The listing builds one solid part. Answer for the finished solid, in the listing's coordinates (mm). Round coordinates to 2 decimals unless told otherwise and drop trailing zeros. Loops run counter-clockwise (first coordinate to the right, second up) from the corner with the lowest first, then second, coordinate; pieces in that order, holes last. Notation, with made-up numbers: (57.25, 11.5) - (102.25, 11.5) arc R19 ccw to (102.25, 41.5) - close; hole circle Ø1 at (52, 51.5). An arc over 180 degrees is marked (long way). One line per item, written item: value.
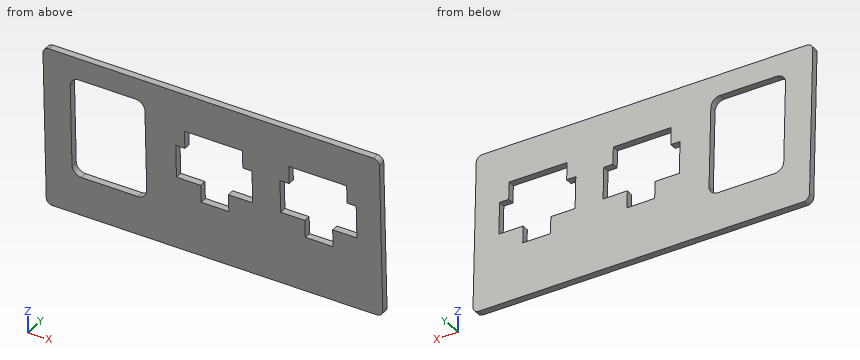
```python
from build123d import *

# Parameters (mm, degrees)
SKETCH1_W           = 110.35
SKETCH1_H           = 52.301351528
BOSS_EXTRUDE1_DEPTH = 2.2
CUT_EXTRUDE1_REACH  = 75.143
FILLET1_R           = 2


with BuildPart() as part:
    # Sketch1 → Boss-Extrude1 (new body)
    with BuildSketch(Plane(origin=(0, -71.98718802, -2.513847999), x_dir=(1, 0, 0), z_dir=(0, 0.9993908270190958, 0.03489949670250105))):
        with Locations((0, 21.739080484)):
            Rectangle(SKETCH1_W, SKETCH1_H)
    extrude(amount=BOSS_EXTRUDE1_DEPTH)

    # Sketch2 → Cut-Extrude1 (cut, up to next)
    with BuildSketch(Plane(origin=(0, -71.98718802, -2.513847999), x_dir=(1, 0, 0), z_dir=(0, -0.9993908270190958, -0.03489949670250106)), mode=Mode.PRIVATE) as cut_extrude1_sk1:
        Polygon((-4.05, -24.262096542), (-4.05, -29.912096542), (5.05, -29.912096542), (5.05, -24.262096542), (13, -24.262096542), (13, -13.662096542), (10, -13.662096542), (10, -7.912096542), (-9, -7.912096542), (-9, -13.662096542), (-12, -13.662096542), (-12, -24.262096542), align=None)
    cut_extrude1_tool1 = extrude(cut_extrude1_sk1.sketch, amount=-CUT_EXTRUDE1_REACH, mode=Mode.PRIVATE) & part.part
    # Sketch2 → Cut-Extrude1 (cut, up to next)
    with BuildSketch(Plane(origin=(0, -71.98718802, -2.513847999), x_dir=(1, 0, 0), z_dir=(0, -0.9993908270190958, -0.03489949670250106)), mode=Mode.PRIVATE) as cut_extrude1_sk2:
        with BuildLine():
            Line((-43.425, -2.662096542), (-24.925, -2.662096542))
            ThreePointArc((-24.925, -2.662096542), (-22.803679656, -3.540776198), (-21.925, -5.662096542))
            Line((-21.925, -5.662096542), (-21.925, -32.162096542))
            ThreePointArc((-21.925, -32.162096542), (-22.803679656, -34.283416885), (-24.925, -35.162096542))
            Line((-24.925, -35.162096542), (-43.425, -35.162096542))
            ThreePointArc((-43.425, -35.162096542), (-45.546320344, -34.283416885), (-46.425, -32.162096542))
            Line((-46.425, -32.162096542), (-46.425, -5.662096542))
            ThreePointArc((-46.425, -5.662096542), (-45.546320344, -3.540776198), (-43.425, -2.662096542))
        make_face()
    cut_extrude1_tool2 = extrude(cut_extrude1_sk2.sketch, amount=-CUT_EXTRUDE1_REACH, mode=Mode.PRIVATE) & part.part
    # Sketch2 → Cut-Extrude1 (cut, up to next)
    with BuildSketch(Plane(origin=(0, -71.98718802, -2.513847999), x_dir=(1, 0, 0), z_dir=(0, -0.9993908270190958, -0.03489949670250106)), mode=Mode.PRIVATE) as cut_extrude1_sk3:
        Polygon((30.125, -24.262096542), (22.175, -24.262096542), (22.175, -13.662096542), (25.175, -13.662096542), (25.175, -7.912096542), (44.175, -7.912096542), (44.175, -13.662096542), (47.175, -13.662096542), (47.175, -24.262096542), (39.225, -24.262096542), (39.225, -29.912096542), (30.125, -29.912096542), align=None)
    cut_extrude1_tool3 = extrude(cut_extrude1_sk3.sketch, amount=-CUT_EXTRUDE1_REACH, mode=Mode.PRIVATE) & part.part
    add(cut_extrude1_tool1.solids().sort_by_distance((0.5, -71.364395, -20.348299))[0], mode=Mode.SUBTRACT)
    add(cut_extrude1_tool2.solids().sort_by_distance((-34.175, -71.327165, -21.414424))[0], mode=Mode.SUBTRACT)
    add(cut_extrude1_tool3.solids().sort_by_distance((34.675, -71.364395, -20.348299))[0], mode=Mode.SUBTRACT)

    # Fillet1
    fillet1_edges = [part.edges().sort_by_distance(p)[0] for p in [
        (-55.175, -69.21652972, -50.336041655),
        (55.175, -69.21652972, -50.336041655),
        (55.175, -71.041820566, 1.933449303),
        (-55.175, -71.041820566, 1.933449303),
    ]]
    fillet(fillet1_edges, radius=FILLET1_R)


solid = part.part
```
1) Each of these flat-tipped pins is pushed along its axis until it touches: pin 1 Ø1.5 at (x, z) = (-27, -38.5) entering from -Y; pin 2 Ø1.5 at (x, y) = (-26.5, -70.5) entering from -Z; pin 3 Ø4 at (x, z) = (-8, -4) entering from -Y. Where does it stop, or does it pass through?
Final values:
pin 1: y = -70.76
pin 2: z = -50.37
pin 3: y = -72.01
2) Consider L1, parallel to X at y = -70.55, z = -10 (3 decimals); L2, parallel to Z at x = -25, y = -71.75; L3, parallel to Y at x = -43, z = 0.5. Determine where each line is inside the solid, lowest interval first.
Final values:
L1: -55.175 to -46.425, -21.925 to 55.175
L2: -5.17 to 1.91
L3: -72.09 to -69.89
3) A cutting plane is placed at B-B on x = -39.5. Give the vertices of the cut face in (y, z).
Final values:
outline: (-72.14, 1.9) - (-71.89, -5.17) - (-69.7, -5.1) - (-69.94, 1.97) - close; (-70.76, -37.65) - (-70.32, -50.37) - (-68.12, -50.3) - (-68.56, -37.58) - close
4) A cutting plane is placed at D-D on z = -45. Give the vertices of the cut face in (x, y) (3 decimals).
Final values:
outline: (-55.175, -70.504) - (55.175, -70.504) - (55.175, -68.302) - (-55.175, -68.302) - close
5) A cutting plane is placed at C-C on z = -18. Give the vertices of the cut face in (x, y) (3 decimals), and give its area (3 significant figures).
Final values:
outline: (-55.175, -71.446) - (-46.425, -71.446) - (-46.425, -69.245) - (-55.175, -69.245) - close; (-21.925, -71.446) - (-12, -71.446) - (-12, -69.245) - (-21.925, -69.245) - close; (13, -71.446) - (22.175, -71.446) - (22.175, -69.245) - (13, -69.245) - close; (47.175, -71.446) - (55.175, -71.446) - (55.175, -69.245) - (47.175, -69.245) - close
area: 78.9 mm2
6) A cutting plane is placed at A-A on x = 8.5. Give the vertices of the cut face in (y, z).
Final values:
outline: (-72.14, 1.9) - (-71.71, -10.42) - (-69.51, -10.34) - (-69.94, 1.97) - close; (-71.14, -26.76) - (-70.32, -50.37) - (-68.12, -50.3) - (-68.94, -26.68) - close
